The listing builds one solid part. Answer for the finished solid, in the listing's coordinates (mm). Face numbers are marked on the shaded views. A direction names the side the tool comes from. Round coordinates to 2 decimals unless told otherwise and drop trailing zeros. Order: outer loops, then holes, each group sorted by start corner. A loop starts at its lowest first (then second) coordinate and runs counter-clockwise, first axis right, second up. Notation, with made-up numbers: (27, 35) -> (40, 35) arc R31 ccw to (40, 64) -> close; hole circle Ø4 at (4, 42.5). An arc over 180 degrees is marked (long way). Return JSON: item names as keys, results as strings. Group by question number.
(1) Determine the mould class of the marked faces 5, 6, 7 and 8 for opening direction X: +X half, -X half, draft (parallel to the pull), parting line (faces both ways), or undercut.
(2) The part is cut by section C-C (z = 6.5). Determine the outline of the cut face in (x, y).
(3) The part is cut by section A-A (x = 0). Determine the outline of the cut face in (y, z), plus the area to 3 significant figures.
(4) Consider line 1 (Z direction, x = -40, y = 6); line 2 (Y direction, x = -10, z = 42); line 3 (X direction, y = 34, z = -29). Determine where each line is inside the solid, lowest interval first. Write a range as [from, to].
(5) The part is cut by section B-B (y = 39.5). Determine the outline of the cut face in (x, z), plus the area to 3 significant figures.
(6) Which of the six approach directions +Z, -Z, +X, -X, +Y, -Y give full straight-line access (tool end or side, diameter ignored) to the marked faces 1, 2, 3 and 4?
(7) The part is cut by section D-D (x = -32.5). Determine the outline of the cut face in (y, z).
(8) Each of these flat-tipped pins is pushed along its axis until it touches: pin 1 (1.9 mm diameter, centred on y = 13, z = 0, fed in from -X); pin 2 (4 mm diameter, centred on y = 10.5, z = 46, fed in from -X); pin 3 (2 mm diameter, centred on x = -38, z = -4, fed in from +Y). Where does it stop, or does it pass through?
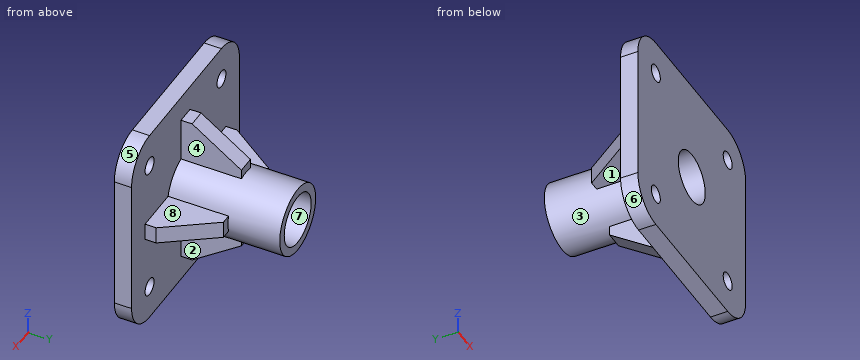
from build123d import *

# Parameters (mm, degrees)
BOSS_EXTRUDE1_DEPTH            = 10
SKETCH2_R                      = 20
BOSS_EXTRUDE2_DEPTH            = 75
BOSS_EXTRUDE3_DEPTH            = 5
CHAMFER1_SIZE                  = 20
CHAMFER1_SIZE2                 = 28.562960134842417
CIRPATTERN1_COUNT              = 4
CHAMFER1_OF_CIRPATTERN1_SIZE2  = 28.562960134842417
CHAMFER1_OF_CIRPATTERN1_SIZE   = 20
SKETCH4_R                      = 15
CUT_EXTRUDE1_DEPTH             = 114.24751652906124
FILLET1_R                      = 20
F_10_0_10_DIAMETER_HOLE1_D     = 10
F_10_0_10_DIAMETER_HOLE1_DEPTH = 10
F_10_0_10_DIAMETER_HOLE1_TIP   = 3.0043030951378014


with BuildPart() as part:
    # Sketch1 → Boss-Extrude1 (new body)
    with BuildSketch(Plane(origin=(0, 0, 0), x_dir=(1, 0, 0), z_dir=(0, 1, 0))):
        Polygon((-60.00000000000001, 59.99999999999999), (59.99999999999999, 59.99999999999999), (60.00000000000001, -60.00000000000001), (-59.99999999999999, -60.00000000000001), align=None)
    extrude(amount=BOSS_EXTRUDE1_DEPTH)

    # Sketch2 → Boss-Extrude2 (add)
    with BuildSketch(Plane.XZ):
        with Locations(Location((0, 0, 0), (0, 0, 270))):
            Circle(SKETCH2_R)
    extrude(amount=-BOSS_EXTRUDE2_DEPTH)

    # Sketch3 → Boss-Extrude3 (add, symmetric)
    with BuildSketch(Plane.XY):
        Polygon((0, 10), (-45, 9.999999999999995), (-45, 45), (0, 45), align=None)
    boss_extrude3 = extrude(amount=BOSS_EXTRUDE3_DEPTH, both=True)

    # Chamfer1
    chamfer1_edges = [part.edges().sort_by_distance(p)[0] for p in [
        (-45, 45, 0),
    ]]
    chamfer1_side = [part.faces().sort_by_distance(p)[0] for p in [
        (-32.39412654979103, 45, 2.29e-15),
    ]]
    chamfer(chamfer1_edges, length=CHAMFER1_SIZE, length2=CHAMFER1_SIZE2, reference=chamfer1_side[0])

    # CirPattern1: Boss-Extrude3 ×4 about axis
    cirpattern1_axis = Axis((-1.07e-15, 0, 7e-17), (0, 1, 0))
    for i in range(1, CIRPATTERN1_COUNT):
        add(boss_extrude3.rotate(cirpattern1_axis, i * 360 / CIRPATTERN1_COUNT))

    # Chamfer1 of CirPattern1
    chamfer1_of_cirpattern1_edges = [part.edges().sort_by_distance(p)[0] for p in [
        (-3.9e-15, 45, 45),
        (45, 45, 5.66e-15),
        (7.27e-15, 45, -45),
    ]]
    chamfer(chamfer1_of_cirpattern1_edges, length=CHAMFER1_OF_CIRPATTERN1_SIZE, length2=CHAMFER1_OF_CIRPATTERN1_SIZE2)

    # Sketch4 → Cut-Extrude1 (cut, through all)
    with BuildSketch(Plane(origin=(0, 75, 0), x_dir=(1, 0, 0), z_dir=(0, 1, 0))):
        with Locations(Location((0, 0, 0), (0, 0, 270))):
            Circle(SKETCH4_R)
    extrude(amount=-CUT_EXTRUDE1_DEPTH, mode=Mode.SUBTRACT)

    # Fillet1
    fillet1_edges = [part.edges().sort_by_distance(p)[0] for p in [
        (60.00000000000001, 5, 60.00000000000001),
        (-59.99999999999999, 5, 60.00000000000001),
        (-60.00000000000001, 5, -59.99999999999999),
        (59.99999999999999, 5, -59.99999999999999),
    ]]
    fillet(fillet1_edges, radius=FILLET1_R)

    # Ø10.0 (10) Diameter Hole1
    with Locations(Plane(origin=(0, 10, 0), x_dir=(-1, 0, 0), z_dir=(0, 1, 0))):
        with Locations((40, -40), (40, 40), (-40, 40), (-40, -40)):
            Hole(F_10_0_10_DIAMETER_HOLE1_D / 2, depth=F_10_0_10_DIAMETER_HOLE1_DEPTH)
            with Locations((0, 0, -(F_10_0_10_DIAMETER_HOLE1_DEPTH + F_10_0_10_DIAMETER_HOLE1_TIP / 2))):  # 118° drill point
                Cone(0, F_10_0_10_DIAMETER_HOLE1_D / 2, F_10_0_10_DIAMETER_HOLE1_TIP, mode=Mode.SUBTRACT)


solid = part.part
Answer below:
{
 "1": {"face 5": "+X half", "face 6": "-X half", "face 7": "undercut", "face 8": "draft"},
 "2": {"outline": "(-60, 0) -> (-13.52, 0) -> (-13.52, 75) -> (-18.91, 75) -> (-18.91, 10) -> (-60, 10) -> close; (13.52, 0) -> (60, 0) -> (60, 10) -> (18.91, 10) -> (18.91, 75) -> (13.52, 75) -> close"},
 "3": {"outline": "(0, -60) -> (10, -60) -> (10, -45) -> (16.44, -45) -> (45, -25) -> (45, -20) -> (75, -20) -> (75, -15) -> (0, -15) -> close; (0, 15) -> (75, 15) -> (75, 20) -> (45, 20) -> (45, 25) -> (16.44, 45) -> (10, 45) -> (10, 60) -> (0, 60) -> close", "area": "2,730 mm²"},
 "4": {"line 1": "z = [-60, -45], [-35, 35], [45, 60]", "line 2": "y = [0, 10]", "line 3": "x = [-5, 5]"},
 "5": {"outline": "(-28.85, -5) -> (-19.36, -5) arc R20 ccw to (-5, -19.36) -> (-5, -28.85) -> (5, -28.85) -> (5, -19.36) arc R20 ccw to (19.36, -5) -> (28.85, -5) -> (28.85, 5) -> (19.36, 5) arc R20 ccw to (5, 19.36) -> (5, 28.85) -> (-5, 28.85) -> (-5, 19.36) arc R20 ccw to (-19.36, 5) -> (-28.85, 5) -> close; hole circle Ø30 at (0, 0)", "area": "912 mm²"},
 "6": {"face 1": "-Z, -X, +Y", "face 2": "-Z, +X, +Y", "face 3": "+Y", "face 4": "+Z, +X, +Y"},
 "7": {"outline": "(0, -60) -> (10, -60) -> (10, -5) -> (34.29, -5) -> (34.29, 5) -> (10, 5) -> (10, 60) -> (0, 60) -> close"},
 "8": {"pin 1": "stops at x = -45", "pin 2": "stops at x = -59.58", "pin 3": "stops at y = 27.86"}
}
